from build123d import *

# Parameters (mm, degrees)
SCHIZZO1_R                   = 1.4
SCHIZZO1_R_2                 = 1.75
ESTRUSIONE_ESTRUSIONE1_DEPTH = 3
SCHIZZO2_R                   = 3.4
SCHIZZO2_R_2                 = 1.4
ESTRUSIONE_ESTRUSIONE2_DEPTH = 3
SCHIZZO3_R                   = 3.8
ESTRUSIONE_ESTRUSIONE3_DEPTH = 15
FORO_2_8_2_8_1_D             = 2.8
FORO_2_8_2_8_1_DEPTH         = 10
SCHIZZO6_W                   = 22.78889745
SCHIZZO6_H                   = 2.4
ESTRUSIONE_ESTRUSIONE4_DEPTH = 8
SMUSSO1_SIZE                 = 1
SCHIZZO8_W                   = 32.32
SCHIZZO8_H                   = 49.15
TAGLIO_ESTRUSIONE1_DEPTH     = 117.922816422


with BuildPart() as part:
    # Schizzo1 → Estrusione-Estrusione1 (new body)
    with BuildSketch(Plane(origin=(0, 0, 0), x_dir=(1, 0, 0), z_dir=(0, 1, 0))):
        with BuildLine():
            Line((-72, 3.636275567), (-72, 81.363724433))
            ThreePointArc((-72, 81.363724433), (-74.019517608, 86.032462202), (-70, 89.15))
            Line((-70, 89.15), (-7.3, 89.15))
            ThreePointArc((-7.3, 89.15), (-3.298340724, 86.09964678), (-5.179319645, 81.432758092))
            Line((-5.179319645, 81.432758092), (-16, 75))
            Line((-16, 75), (-16, 20))
            Line((-16, 20), (2.777722531, 3.083303025))
            ThreePointArc((2.777722531, 3.083303025), (3.87415846, -1.48774871), (0, -4.15))
            Line((0, -4.15), (-70, -4.15))
            ThreePointArc((-70, -4.15), (-74.019517608, -1.032462202), (-72, 3.636275567))
        make_face()
        with Locations(Location((-67.82, 12.25, 0), (0, 0, 270))):
            Circle(SCHIZZO1_R, mode=Mode.SUBTRACT)
        with Locations(Location((-19.5, 11, 0), (0, 0, 270))):
            Circle(SCHIZZO1_R, mode=Mode.SUBTRACT)
        with Locations(Location((-24.32, 63, 0), (0, 0, 270))):
            Circle(SCHIZZO1_R, mode=Mode.SUBTRACT)
        with Locations(Location((-52.49, 63, 0), (0, 0, 270))):
            Circle(SCHIZZO1_R, mode=Mode.SUBTRACT)
        with Locations(Location((0, 0, 0), (0, 0, 270))):
            Circle(SCHIZZO1_R_2, mode=Mode.SUBTRACT)
        with Locations(Location((-70, 0, 0), (0, 0, 270))):
            Circle(SCHIZZO1_R_2, mode=Mode.SUBTRACT)
        with Locations(Location((-70, 85, 0), (0, 0, 270))):
            Circle(SCHIZZO1_R_2, mode=Mode.SUBTRACT)
        with Locations(Location((-7.3, 85, 0), (0, 0, 270))):
            Circle(SCHIZZO1_R_2, mode=Mode.SUBTRACT)
    extrude(amount=ESTRUSIONE_ESTRUSIONE1_DEPTH)

    # Schizzo2 → Estrusione-Estrusione2 (add)
    # profile 1 of 4: a face of its own
    with BuildSketch(Plane(origin=(0, 3, 0), x_dir=(1, 0, 0), z_dir=(0, 1, 0))):
        with Locations(Location((-67.82, 12.25, 0), (0, 0, 270))):
            Circle(SCHIZZO2_R)
        with Locations(Location((-67.82, 12.25, 0), (0, 0, 270))):
            Circle(SCHIZZO2_R_2, mode=Mode.SUBTRACT)
    # profile 2 of 4: a face of its own
    with BuildSketch(Plane(origin=(0, 3, 0), x_dir=(1, 0, 0), z_dir=(0, 1, 0))):
        with Locations(Location((-19.5, 11, 0), (0, 0, 270))):
            Circle(SCHIZZO2_R)
        with Locations(Location((-19.5, 11, 0), (0, 0, 270))):
            Circle(SCHIZZO2_R_2, mode=Mode.SUBTRACT)
    # profile 3 of 4: a face of its own
    with BuildSketch(Plane(origin=(0, 3, 0), x_dir=(1, 0, 0), z_dir=(0, 1, 0))):
        with Locations(Location((-24.32, 63, 0), (0, 0, 270))):
            Circle(SCHIZZO2_R)
        with Locations(Location((-24.32, 63, 0), (0, 0, 270))):
            Circle(SCHIZZO2_R_2, mode=Mode.SUBTRACT)
    # profile 4 of 4: a face of its own
    with BuildSketch(Plane(origin=(0, 3, 0), x_dir=(1, 0, 0), z_dir=(0, 1, 0))):
        with Locations(Location((-52.49, 63, 0), (0, 0, 270))):
            Circle(SCHIZZO2_R)
        with Locations(Location((-52.49, 63, 0), (0, 0, 270))):
            Circle(SCHIZZO2_R_2, mode=Mode.SUBTRACT)
    extrude(amount=ESTRUSIONE_ESTRUSIONE2_DEPTH)

    # Schizzo3 → Estrusione-Estrusione3 (add)
    with BuildSketch(Plane(origin=(0, 3, 0), x_dir=(1, 0, 0), z_dir=(0, 1, 0))):
        with Locations(Location((-61.5, 79.15, 0), (0, 0, 270))):
            Circle(SCHIZZO3_R)
        with Locations(Location((-31.5, 79.15, 0), (0, 0, 270))):
            Circle(SCHIZZO3_R)
    extrude(amount=ESTRUSIONE_ESTRUSIONE3_DEPTH)

    # Foro Ø2.8 (2.8)-1
    with Locations(Plane(origin=(0, 18, 0), x_dir=(1, 0, 0), z_dir=(0, 1, 0))):
        with Locations((-61.5, 79.15), (-31.5, 79.15)):
            Hole(FORO_2_8_2_8_1_D / 2, depth=FORO_2_8_2_8_1_DEPTH)

    # Schizzo6 → Estrusione-Estrusione4 (add)
    with BuildSketch(Plane(origin=(0, 3, 0), x_dir=(1, 0, 0), z_dir=(0, 1, 0))):
        with Locations((-46.5, 79.15)):
            Rectangle(SCHIZZO6_W, SCHIZZO6_H)
    extrude(amount=ESTRUSIONE_ESTRUSIONE4_DEPTH)

    # Smusso1
    smusso1_edges = [part.edges().sort_by_distance(p)[0] for p in [
        (-28.417792999, 3, -81.372611077),
        (-64.582207001, 3, -81.372611077),
    ]]
    chamfer(smusso1_edges, length=SMUSSO1_SIZE)

    # Schizzo8 → Taglio-Estrusione1 (cut, through all)
    with BuildSketch(Plane(origin=(0, 3, 0), x_dir=(1, 0, 0), z_dir=(0, 1, 0))):
        with Locations((-43.66, 30.425)):
            Rectangle(SCHIZZO8_W, SCHIZZO8_H)
    extrude(amount=-TAGLIO_ESTRUSIONE1_DEPTH, mode=Mode.SUBTRACT)


solid = part.part
Here's how the part is built. I have some questions about the finished solid (model axes, mm). A direction names the side the tool comes from. Round coordinates to 2 decimals unless told otherwise and drop trailing zeros. Loops run counter-clockwise (first coordinate to the right, second up) from the corner with the lowest first, then second, coordinate; pieces in that order, holes last.
1. We'd pull the mould along Z, two halves only. Please class faces 4 (the face through (-22.82, 4.48, -11.74)), 5 (the face through (-47, 7, -80.35)), 6 (the face through (-20.2, 6, -9.5)): +Z half, -Z half, draft (parallel to the pull), parting line (faces both ways), or undercut.
Answer list:
face 4: undercut
face 5: -Z half
face 6: draft
2. If we section it at A-A on y = 5: Count the separate pieces of the cut face and the enclosed holes in it, plus the area to 3 significant figures.
Answer list:
separate pieces: 5
enclosed holes: 4
area: 265 mm2
3. Which directions (+Z, -Z, +X, -X, +Y, -Y) give clear straight access to the entire face, cutting with the end or side of a thin tool? Please do faces 1 (the face through (-25.62, 4.48, -59.86)), 2 (the face through (-16, 1, -48)), 3 (the face through (-26, 0, -43)).
Answer list:
face 1: +Y
face 2: +X, +Y, -Y
face 3: +Z, -Z, +X, -X, -Y
4. If we section it at B-B on x = -19.5: Write out the boundary of the cut face in (y, z).
Answer list:
outline: (0, -89.15) - (3, -89.15) - (3, -14.4) - (6, -14.4) - (6, -12.4) - (0, -12.4) - close; (0, -9.6) - (6, -9.6) - (6, -7.6) - (3, -7.6) - (3, 4.15) - (0, 4.15) - close
5. If I drill on line 1 along X through (y, z) = (12.25, -79.15); line 2 along X through (y, z) = (1.25, 0); line 3 along Z through (x, y) = (-70, 1.55), over which ranges is the centre line in solid material (lowest first)?
Answer list:
line 1: x = -65.3 to -62.9, -60.1 to -57.7, -35.3 to -32.9, -30.1 to -27.7
line 2: x = -74.15 to -71.75, -68.25 to -1.75, 1.75 to 4.15
line 3: z = -89.15 to -86.75, -83.25 to -1.75, 1.75 to 4.15
6. For P1, Ø3, axis at x = -61, z = -79, coming from the +Y side; P2, Ø2, axis at x = -70, z = 0, coming from the -Y side; P3, Ø1, axis at x = -26.5, z = -41.5, coming from the +Y side; P4, Ø3.5, axis at x = -24.5, z = -61.5, coming from the +Y side, each with a flat end and sliding along its axis, tell me the tip position at first contact or that it passes through.
Answer list:
P1: stops at y = 18
P2: passes through
P3: stops at y = 3
P4: stops at y = 6
7. If we section it at C-C on z = -54: Write out the boundary of the cut face in (x, y).
Answer list:
outline: (-72, 0) - (-59.82, 0) - (-59.82, 3) - (-72, 3) - close; (-27.5, 0) - (-16, 0) - (-16, 3) - (-27.5, 3) - close
8. If we section it at D-D on y = 15.5: Write out the boundary of the cut face in (x, z), plus the area to 3 significant figures.
Answer list:
outline: circle Ø7.6 at (-61.5, -79.15); circle Ø7.6 at (-31.5, -79.15); hole circle Ø2.8 at (-61.5, -79.15); hole circle Ø2.8 at (-31.5, -79.15)
area: 78.4 mm2
